from build123d import *

# Parameters (mm, degrees)
P_IDAT_VYSUNUT_M1_DEPTH = 21.8
ZAOBLIT1_R              = 1
SKICA2_R                = 0.4
P_IDAT_VYSUNUT_M2_DEPTH = 4


with BuildPart() as part:
    # Skica1 → Přidat vysunutím1 (new body)
    with BuildSketch(Plane.XY):
        with BuildLine():
            Line((1, 0), (31.8, 0))
            ThreePointArc((31.8, 0), (32.507106781, 0.292893219), (32.8, 1))
            Line((32.8, 1), (32.8, 26.8))
            ThreePointArc((32.8, 26.8), (32.507106781, 27.507106781), (31.8, 27.8))
            Line((31.8, 27.8), (1, 27.8))
            ThreePointArc((1, 27.8), (0.292893219, 27.507106781), (0, 26.8))
            Line((0, 26.8), (0, 1))
            ThreePointArc((0, 1), (0.292893219, 0.292893219), (1, 0))
        make_face()
    extrude(amount=P_IDAT_VYSUNUT_M1_DEPTH)

    # Zaoblit1
    zaoblit1_edges = [part.edges().sort_by_distance(p)[0] for p in [
        (32.507106781, 27.507106781, 21.8),
        (16.4, 27.8, 21.8),
        (0.292893219, 27.507106781, 21.8),
        (0, 13.9, 21.8),
        (0.292893219, 0.292893219, 21.8),
        (16.4, 0, 21.8),
        (32.507106781, 0.292893219, 21.8),
        (32.8, 13.9, 21.8),
    ]]
    fillet(zaoblit1_edges, radius=ZAOBLIT1_R)

    # Skica2 → Přidat vysunutím2 (add)
    with BuildSketch(Plane.XY):
        with Locations((21.4, 3.9)):
            Circle(SKICA2_R)
        with Locations((26.4, 23.9)):
            Circle(SKICA2_R)
        with Locations((6.4, 23.9)):
            Circle(SKICA2_R)
        with Locations((11.4, 3.9)):
            Circle(SKICA2_R)
    extrude(amount=-P_IDAT_VYSUNUT_M2_DEPTH)


solid = part.part
Here's how the part is built. I have some questions about the finished solid (model axes, mm). A direction names the side the tool comes from. Give positions to 0.01 mm unless a question says otherwise; leave off trailing zeros. Order: outer loops, then holes, each group sorted by start corner. A loop starts at its lowest first (then second) coordinate and runs counter-clockwise, first axis right, second up. Notation, with made-up numbers: M -31,51.5 L 16,51.5 A19 ccw 16,71.5 Z; hole C 40,-4 d1. An arc over 180 degrees is marked long. Answer as a JSON object with one key per item and string values. Group by question number.
1) Please list where this line runs through material, in increasing order: L1, parallel to Z at x = 11.5, y = 26.25. Write a range as [from, to].
2) On a 3-axis mill with a long thin cutter (end or side, diameter ignored), from which of +Z, -Z, +X, -X, +Y, -Y can I reach the whole of each face in a straight line? I mean faces 1 (the cylindrical face through (0.301, 27.515, 10.254)), 2 (the cylindrical face through (11.08, 3.66, -1.97)). Say none if no direction works.
3) Suppose I cut it at C-C, the plane x = 14. Write out the boundary of the cut face in (y, z), plus the area to 3 significant figures.
4) Suppose I cut it at A-A, the plane y = 14. Write out the boundary of the cut face in (x, z).
5) Suppose I cut it at B-B, the plane z = -1.5. Write out the boundary of the cut face in (x, y).
Results found:
{
 "1": {"L1": "[0, 21.8]"},
 "2": {"face 1": "+Z, -Z, -X, +Y", "face 2": "-Z"},
 "3": {"outline": "M 0,0 L 27.8,0 L 27.8,20.8 A1 ccw 26.8,21.8 L 1,21.8 A1 ccw 0,20.8 Z", "area": "606 mm²"},
 "4": {"outline": "M 0,0 L 32.8,0 L 32.8,20.8 A1 ccw 31.8,21.8 L 1,21.8 A1 ccw 0,20.8 Z"},
 "5": {"outline": "C 6.4,23.9 d0.8; C 11.4,3.9 d0.8; C 21.4,3.9 d0.8; C 26.4,23.9 d0.8"}
}
